from build123d import *

# Parameters (mm, degrees)
REVOLUCI_N_L_MINA1_ANGLE      = 180
CORTAR_EXTRUIR1_START         = -10
CORTAR_EXTRUIR1_DEPTH         = 100
CORTAR_EXTRUIR2_DEPTH         = 184
CORTAR_EXTRUIR2_DEPTH_BACK    = 4
CROQUIS4_W                    = 20
CROQUIS4_H                    = 10
TALADRO_ROSCADO_M4X0_71_D     = 3.3
TALADRO_ROSCADO_M4X0_71_DEPTH = 12
TALADRO_ROSCADO_M4X0_71_TIP   = 0.991420021


with BuildPart() as part:
    # Croquis1 → Revolución-Lámina1 (revolve)
    with BuildSketch(Plane(origin=(0, 0, 0), x_dir=(1, 0, 0), z_dir=(0, 1, 0))):
        with BuildLine():
            ThreePointArc((0, 100), (100, 0), (0, -100))
            Line((0, -100), (0, -90))
            ThreePointArc((0, -90), (90, 0), (0, 90))
            Line((0, 90), (0, 100))
        make_face()
    revolve(axis=Axis((0, 0, -100), (0, 0, -1)), revolution_arc=REVOLUCI_N_L_MINA1_ANGLE)

    # Croquis2 → Cortar-Extruir1 (cut)
    with BuildSketch(Plane(origin=(0, 0, 0), x_dir=(1, 0, 0), z_dir=(0, 1, 0)).offset(CORTAR_EXTRUIR1_START)):
        Polygon((17.5, 30.310889132), (-17.5, 30.310889132), (-35, 0), (-17.5, -30.310889132), (17.5, -30.310889132), (35, 0), align=None)
        Polygon((104.820508076, 40.310889132), (87.320508076, 70.621778265), (52.320508076, 70.621778265), (34.820508076, 40.310889132), (52.320508076, 10), (87.320508076, 10), align=None)
        Polygon((17.5, 110.932667397), (-17.5, 110.932667397), (-35, 80.621778265), (-17.5, 50.310889132), (17.5, 50.310889132), (35, 80.621778265), align=None)
        Polygon((87.320508076, -70.621778265), (104.820508076, -40.310889132), (87.320508076, -10), (52.320508076, -10), (34.820508076, -40.310889132), (52.320508076, -70.621778265), align=None)
        Polygon((-17.5, -110.932667397), (17.5, -110.932667397), (35, -80.621778265), (17.5, -50.310889132), (-17.5, -50.310889132), (-35, -80.621778265), align=None)
        Polygon((-104.820508076, -40.310889132), (-87.320508076, -70.621778265), (-52.320508076, -70.621778265), (-34.820508076, -40.310889132), (-52.320508076, -10), (-87.320508076, -10), align=None)
        Polygon((-87.320508076, 70.621778265), (-104.820508076, 40.310889132), (-87.320508076, 10), (-52.320508076, 10), (-34.820508076, 40.310889132), (-52.320508076, 70.621778265), align=None)
    extrude(amount=-CORTAR_EXTRUIR1_DEPTH, mode=Mode.SUBTRACT)

    # Croquis4 → Cortar-Extruir2 (cut, two sides: drawn at the far end of the back side and taken through both)
    with BuildSketch(Plane.ZY.offset(-90).offset(-CORTAR_EXTRUIR2_DEPTH_BACK)):
        Rectangle(CROQUIS4_W, CROQUIS4_H)
    extrude(amount=CORTAR_EXTRUIR2_DEPTH + CORTAR_EXTRUIR2_DEPTH_BACK, mode=Mode.SUBTRACT)

    # Taladro roscado M4x0.71
    with Locations(Plane(origin=(0, 0, 0), x_dir=(1, 0, 0), z_dir=(0, 1, 0))):
        with Locations((-47.5, -82.27241336), (47.5, 82.27241336), (47.5, -82.27241336), (-47.5, 82.27241336)):
            Hole(TALADRO_ROSCADO_M4X0_71_D / 2, depth=TALADRO_ROSCADO_M4X0_71_DEPTH)
            with Locations((0, 0, -(TALADRO_ROSCADO_M4X0_71_DEPTH + TALADRO_ROSCADO_M4X0_71_TIP / 2))):  # 118° drill point
                Cone(0, TALADRO_ROSCADO_M4X0_71_D / 2, TALADRO_ROSCADO_M4X0_71_TIP, mode=Mode.SUBTRACT)


solid = part.part
Read the model definition and answer for the solid it produces. Units are mm, in the model's axes. A direction names the side the tool comes from. Round coordinates to 2 decimals unless told otherwise and drop trailing zeros. Order: outer loops, then holes, each group sorted by start corner. A loop starts at its lowest first (then second) coordinate and runs counter-clockwise, first axis right, second up. Notation, with made-up numbers: (78, 87) - (106, 87) arc R25 cw to (106, 117) - close; hole circle Ø3 at (17, 82). An arc over 180 degrees is marked (long way). Use one line per item in the form item = value. Start each with the question number.
(1) Find the intervals of material crossed by line 1 along Z through (x, y) = (9.5, -85.5); line 2 along Z through (x, y) = (-47, -5); line 3 along Z through (x, y) = (47, -9), in increasing order. Write a range as from..to.
(2) Determine the mould class of faces 1 (the face through (44.826, -59.099, 57.641)), 2 (the face through (-90.713, -24.397, 15.877)), 3 (the face through (26.372, -89.019, -14.943)), 4 (the face through (-72, -59, -10)) for opening direction Z: +Z half, -Z half, draft (parallel to the pull), parting line (faces both ways), or undercut.
(3) The part is cut by section A-A (x = -40). Give the vertices of the cut face in (y, z).
(4) The part is cut by section C-C (y = -55.5). Give the vertices of the cut face in (x, z).
(5) For faces 5 (the face through (92, -3, -10)), 6 (the face through (-90.838, -24.397, -16.092)), 7 (the face through (59, -24, -70.622)), 8 (the face through (-59, -24, 70.622)), determine the directions among +Z, -Z, +X, -X, +Y, -Y from which every point of the face is accessible in a straight line to the end or side of a thin tool.
(6) Flat-ended cylindrical pins translate along their axes: pin 1 Ø1.4 at (x, y) = (92.5, -2.5) entering from -Z; pin 2 Ø2.5 at (x, y) = (-91, -2) entering from -Z; pin 3 Ø1 at (y, z) = (-44.5, 77) entering from -X. Find the tip coordinate at first contact, or state that the pin passes through.
(7) The part is cut by section D-D (x = 12). Give the vertices of the cut face in (y, z).
(8) The part is cut by section B-B (z = -65.5). Give the vertices of the cut face in (x, y).
Checked values:
q1.line_1 = -50.31..-30.31, 30.31..50.31
q1.line_2 = -88.12..-83.84, -80.7..-76.59, 76.59..80.7, 83.84..88.12
q1.line_3 = -87.81..-83.84, -80.7..-76.22, 76.22..80.7, 83.84..87.81
q2.face_1 = undercut
q2.face_2 = +Z half
q2.face_3 = undercut
q2.face_4 = -Z half
q3.outline = (-86.13, -31.34) - (-74.28, -31.34) arc R80.62 cw to (-74.28, 31.34) - (-86.13, 31.34) arc R91.65 ccw to start; (-77.27, -49.28) arc R91.65 ccw to (0, -91.65) - (0, -80.62) arc R80.62 cw to (-63.81, -49.28) - close; (-77.27, 49.28) - (-63.81, 49.28) arc R80.62 cw to (0, 80.62) - (0, 91.65) arc R91.65 ccw to start
q4.outline = (-82.58, -10) - (-70.14, -10) arc R70.85 cw to (-70.14, 10) - (-82.58, 10) arc R83.19 ccw to start; (-49.95, -66.52) arc R83.19 ccw to (-32.63, -76.52) - (-26.41, -65.74) arc R70.85 cw to (-43.73, -55.74) - close; (-49.95, 66.52) - (-43.73, 55.74) arc R70.85 cw to (-26.41, 65.74) - (-32.63, 76.52) arc R83.19 ccw to start; (26.41, -65.74) - (32.63, -76.52) arc R83.19 ccw to (49.95, -66.52) - (43.73, -55.74) arc R70.85 cw to start; (26.41, 65.74) arc R70.85 cw to (43.73, 55.74) - (49.95, 66.52) arc R83.19 ccw to (32.63, 76.52) - close; (70.14, -10) - (82.58, -10) arc R83.19 ccw to (82.58, 10) - (70.14, 10) arc R70.85 cw to start
q5.face_5 = +Y
q5.face_6 = -Z, -Y
q5.face_7 = +X, -Y
q5.face_8 = -X, -Y
q6.pin_1 = -39.58
q6.pin_2 = -44.06
q6.pin_3 = -46.68
q7.outline = (-94.54, -30.31) arc R99.28 ccw to (-85.59, -50.31) - (-73.65, -50.31) arc R89.2 cw to (-83.89, -30.31) - close; (-94.54, 30.31) - (-83.89, 30.31) arc R89.2 cw to (-73.65, 50.31) - (-85.59, 50.31) arc R99.28 ccw to start; (-10, -98.77) arc R99.28 ccw to (0, -99.28) - (0, -89.2) arc R89.2 cw to (-10, -88.63) - close; (-10, 88.63) arc R89.2 cw to (0, 89.2) - (0, 99.28) arc R99.28 ccw to (-10, 98.77) - close
q8.outline = (-75.56, 0) arc R75.56 ccw to (-74.9, -10) - (-60.91, -10) arc R61.72 cw to (-61.72, 0) - close; (-49.36, -57.21) arc R75.56 ccw to (-26.27, -70.85) - (-26.27, -55.85) arc R61.72 cw to (-49.36, -37.05) - close; (26.27, -70.85) arc R75.56 ccw to (49.36, -57.21) - (49.36, -37.05) arc R61.72 cw to (26.27, -55.85) - close; (60.91, -10) - (74.9, -10) arc R75.56 ccw to (75.56, 0) - (61.72, 0) arc R61.72 cw to start
